Work out the finished part from the listing and answer in its coordinate system (mm). Face numbers are marked on the shaded views. A direction names the side the tool comes from. Round coordinates to 2 decimals unless told otherwise and drop trailing zeros. Order: outer loops, then holes, each group sorted by start corner. A loop starts at its lowest first (then second) coordinate and runs counter-clockwise, first axis right, second up. Notation, with made-up numbers: (-35, 31.25) - (23, 31.25) arc R15 cw to (23, 52.25) - close; hole circle Ø4 at (47, -11.75). An arc over 180 degrees is marked (long way). Put each result on its own line as item: value.
```python
from build123d import *

# Parameters (mm, degrees)
F0_W      = 69.85
F0_H      = 44.45
F1_DEPTH  = 3.175
F2_W      = 69.85
F2_H      = 44.45
F2_W_2    = 63.5
F2_H_2    = 38.1
F3_DEPTH  = 25.4
F4_W      = 69.85
F4_H      = 3.175
F5_DEPTH  = 6.223
F6_W      = 69.85
F6_H      = 3.048
F7_DEPTH  = 3.048
F8_W      = 69.85
F8_H      = 3.048
F9_DEPTH  = 3.048
F10_W     = 63.5
F10_H     = 3.175
F11_DEPTH = 3.175
F12_W     = 63.5
F12_H     = 3.175
F13_DEPTH = 3.175
F14_W     = 31.75
F14_H     = 3.175
F15_DEPTH = 3.175
F16_W     = 3.302
F16_H     = 6.223
F17_DEPTH = 38.1


with BuildPart() as f1:
    # F0 (on Top) → F1 (new body)
    with BuildSketch(Plane.XY):
        with Locations((34.925, 22.225)):
            Rectangle(F0_W, F0_H)
    extrude(amount=F1_DEPTH)

    # F2 (on face) → F3 (join)
    with BuildSketch(Plane.XY.offset(3.175)):
        with Locations((34.925, 22.225)):
            Rectangle(F2_W, F2_H)
        with Locations((34.925, 22.225)):
            Rectangle(F2_W_2, F2_H_2, mode=Mode.SUBTRACT)
    extrude(amount=F3_DEPTH)

    # F4 (on face) → F5 (join)
    with BuildSketch(Plane(origin=(0, 0, 0), x_dir=(1, 0, 0), z_dir=(0, 0, -1))):
        with Locations((34.925, -8.0645)):
            Rectangle(F4_W, F4_H)
        with Locations((34.925, -36.3855)):
            Rectangle(F4_W, F4_H)
    extrude(amount=F5_DEPTH)

    # F6 (on face) → F7 (join)
    with BuildSketch(Plane.XZ.offset(-6.477)):
        with Locations((34.925, -4.699)):
            Rectangle(F6_W, F6_H)
    extrude(amount=F7_DEPTH)

    # F8 (on face) → F9 (join)
    with BuildSketch(Plane(origin=(0, 37.973, 0), x_dir=(-1, 0, 0), z_dir=(0, 1, 0))):
        with Locations((-34.925, -4.699)):
            Rectangle(F8_W, F8_H)
    extrude(amount=F9_DEPTH)

    # F10 (on face) → F11 (join)
    with BuildSketch(Plane(origin=(0, 3.175, 0), x_dir=(-1, 0, 0), z_dir=(0, 1, 0))):
        with Locations((-34.925, 26.9875)):
            Rectangle(F10_W, F10_H)
    extrude(amount=F11_DEPTH)

    # F12 (on face) → F13 (join)
    with BuildSketch(Plane.XZ.offset(-41.275)):
        with Locations((34.925, 26.9875)):
            Rectangle(F12_W, F12_H)
    extrude(amount=F13_DEPTH)

    # F14 (on face) → F15 (cut, through all)
    with BuildSketch(Plane.YZ.offset(69.85)):
        Polygon((38.1, 25.4), (6.35, 25.4), (3.175, 25.4), (3.175, 22.225), (41.275, 22.225), (41.275, 25.4), align=None)
        with Locations((22.225, 26.9875)):
            Rectangle(F14_W, F14_H)
    extrude(amount=-F15_DEPTH, mode=Mode.SUBTRACT)

    # F16 (on face) → F17 (cut)
    with BuildSketch(Plane.XZ.offset(-3.429)):
        with Locations((1.651, -3.1115)):
            Rectangle(F16_W, F16_H)
    extrude(amount=-F17_DEPTH, mode=Mode.SUBTRACT)


solid = f1.part
```
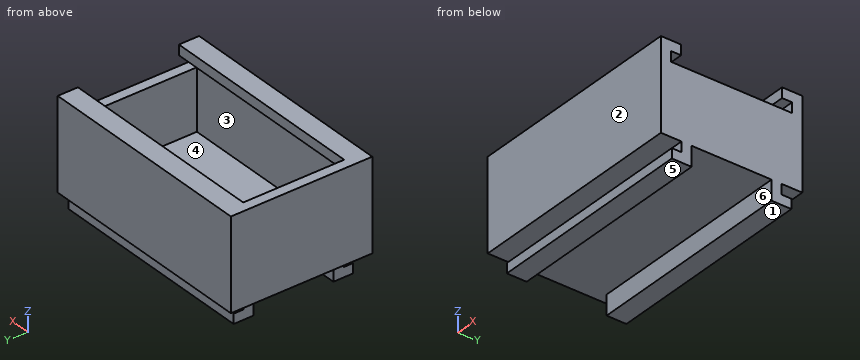
1) A cutting plane is placed at D-D on z = 23. Write down the section's boundary in (x, y) (3 decimals).
Findings below:
outline: (0, 0) - (69.85, 0) - (69.85, 3.175) - (3.175, 3.175) - (3.175, 41.275) - (69.85, 41.275) - (69.85, 44.45) - (0, 44.45) - close
2) Straight lines are drawn through the part: L1, parallel to Z at x = 35.5, y = 39 (3 decimals); L2, parallel to X at y = 40.5, z = 8 (3 decimals); L3, parallel to Y at x = 66, z = 23 (3 decimals). For each, find the intervals that lie inside material, in ascending order. Write a range as from..to.
Findings below:
L1: z = -6.223..-3.175, 0..3.175, 25.4..28.575
L2: x = 0..3.175, 66.675..69.85
L3: y = 0..3.175, 41.275..44.45
3) A cutting plane is placed at A-A on z = -2. Write down the section's boundary in (x, y).
Findings below:
outline: (3.3, 6.48) - (69.85, 6.48) - (69.85, 9.65) - (3.3, 9.65) - close; (3.3, 34.8) - (69.85, 34.8) - (69.85, 37.97) - (3.3, 37.97) - close
4) A cutting plane is placed at C-C on x = 27. Write down the section's boundary in (y, z) (3 decimals).
Findings below:
outline: (0, 0) - (6.477, 0) - (6.477, -3.175) - (3.429, -3.175) - (3.429, -6.223) - (9.652, -6.223) - (9.652, 0) - (34.798, 0) - (34.798, -6.223) - (41.021, -6.223) - (41.021, -3.175) - (37.973, -3.175) - (37.973, 0) - (44.45, 0) - (44.45, 28.575) - (38.1, 28.575) - (38.1, 25.4) - (41.275, 25.4) - (41.275, 3.175) - (3.175, 3.175) - (3.175, 25.4) - (6.35, 25.4) - (6.35, 28.575) - (0, 28.575) - close
5) Given pin 1 Ø3.5 at (x, z) = (39, -2) entering from -Y; pin 2 Ø1.9 at (y, z) = (36.5, -4.5) entering from -X; pin 3 Ø2 at (x, y) = (31.5, 25) entering from -Z, each flat-ended and moving along its own axis, determine where each tip first touches the part or whether it passes through.
Findings below:
pin 1: stops at y = 3.43
pin 2: stops at x = 3.3
pin 3: stops at z = 0
6) For the marked faces 4, 5 and 6, determine the directions among +Z, -Z, +X, -X, +Y, -Y from which every point of the face is accessible in a straight line to the end or side of a thin tool.
Findings below:
face 4: none
face 5: -Z, +X, -X, +Y, -Y
face 6: -Z, +X, -X
7) A cutting plane is placed at B-B on y = 31.5. Write down the section's boundary in (x, z) (3 decimals), then the cut area to 3 significant figures.
Findings below:
outline: (0, 0) - (69.85, 0) - (69.85, 22.225) - (66.675, 22.225) - (66.675, 3.175) - (3.175, 3.175) - (3.175, 28.575) - (0, 28.575) - close
area: 363 mm2
8) For a pull along Z with two mould halves and no side action, classify the marked faces 1, 2 and 3 as pulls with the +Z half, pulls with the -Z half, needs draft (parallel to the pull), parting line crosses it, or undercut.
Findings below:
face 1: pulls with the -Z half
face 2: needs draft
face 3: undercut
